Design review of the part built by this model. Coordinates are the model's own, in mm. Give positions to 0.01 mm unless a question says otherwise; leave off trailing zeros. Write each loop counter-clockwise with the first axis right and the second up, starting at its lowest first coordinate (ties: lowest second). Pieces come first, ordered by that corner, then holes. Notation, with made-up numbers: (-3.5, -24.75) -> (23.5, -24.75) arc R16 ccw to (23.5, -7.75) -> close; hole circle Ø3 at (17, 70.5). An arc over 180 degrees is marked (long way). Return JSON: item names as keys, results as strings. Group by question number.
from build123d import *

# Parameters (mm, degrees)
SKETCH1_W                       = 66.04
SKETCH1_H                       = 15.24
BOSS_EXTRUDE1_DEPTH             = 6
CBORE_FOR_M3_SBHCS1_D           = 3.6
CBORE_FOR_M3_SBHCS1_CBORE_D     = 6.7
CBORE_FOR_M3_SBHCS1_CBORE_DEPTH = 1.65
FILLET1_R                       = 5.08
FILLET2_R                       = 1.27


with BuildPart() as part:
    # Sketch1 → Boss-Extrude1 (new body)
    with BuildSketch(Plane(origin=(0, 0, 0), x_dir=(1, 0, 0), z_dir=(0, 1, 0))):
        with Locations((33.02, -7.62)):
            Rectangle(SKETCH1_W, SKETCH1_H)
    extrude(amount=BOSS_EXTRUDE1_DEPTH)

    # CBORE for M3 SBHCS1 (through all)
    with Locations(Plane(origin=(0, 6, 0), x_dir=(1, 0, 0), z_dir=(0, 1, 0))):
        with Locations((16.51, -7.62), (49.53, -7.62)):
            CounterBoreHole(CBORE_FOR_M3_SBHCS1_D / 2, CBORE_FOR_M3_SBHCS1_CBORE_D / 2, CBORE_FOR_M3_SBHCS1_CBORE_DEPTH)

    # Fillet1
    fillet1_edges = [part.edges().sort_by_distance(p)[0] for p in [
        (0, 3, 0),
        (66.04, 3, 0),
        (66.04, 3, 15.24),
        (0, 3, 15.24),
    ]]
    fillet(fillet1_edges, radius=FILLET1_R)

    # Fillet2
    fillet2_edges = [part.edges().sort_by_distance(p)[0] for p in [
        (33.02, 6, 15.24),
        (0, 6, 7.62),
        (66.04, 6, 7.62),
        (33.02, 6, 0),
        (64.552102448, 6, 1.487897552),
        (64.552102448, 6, 13.752102448),
        (1.487897552, 6, 1.487897552),
        (1.487897552, 6, 13.752102448),
    ]]
    fillet(fillet2_edges, radius=FILLET2_R)


solid = part.part
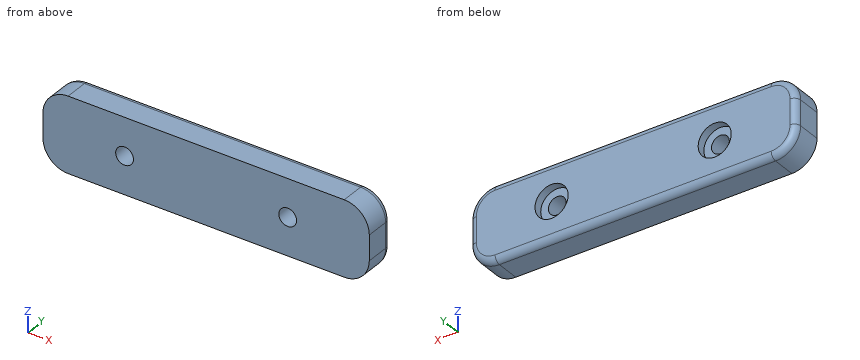
Q1. Take a section at B-B, the plane x = 49.53. Give the boundary of the cut face in (y, z), plus the area to 3 significant figures.
Q2. Insertion check: pin 1 (3.5 mm diameter, centred on x = 16.5, z = 9, fed in from +Y); pin 2 (1.5 mm diameter, centred on y = 2, z = 13.5, fed in from -X). Each pin has a flat end and moves straight along its axis. Give the tip position at first contact, or say it passes through.
Q3. For L1, parallel to X at y = 1.3, z = 7.62; L2, parallel to X at y = 5.6, z = 10; L3, parallel to Z at x = 49.53, y = 5, list the stretches that pass through material, from the lowest coordinate up. Write a range as from..to.
Q4. Take a section at A-A, the plane z = 7.62. Give the boundary of the cut face in (x, y).
Q5. Take a section at C-C, the plane y = 3.65. Give the boundary of the cut face in (x, z).
Final values:
{
 "1": {"outline": "(0, 0) -> (4.73, 0) arc R1.27 ccw to (6, 1.27) -> (6, 4.27) -> (4.35, 4.27) -> (4.35, 5.82) -> (0, 5.82) -> close; (0, 9.42) -> (4.35, 9.42) -> (4.35, 10.97) -> (6, 10.97) -> (6, 13.97) arc R1.27 ccw to (4.73, 15.24) -> (0, 15.24) -> close", "area": "64.0 mm²"},
 "2": {"pin 1": "stops at y = 4.35", "pin 2": "stops at x = 0.71"},
 "3": {"L1": "x = 0..14.71, 18.31..47.73, 51.33..66.04", "L2": "x = 0.34..14.15, 18.87..47.17, 51.89..65.7", "L3": "z = 0.03..4.27, 10.97..15.21"},
 "4": {"outline": "(0, 0) -> (14.71, 0) -> (14.71, 4.35) -> (13.16, 4.35) -> (13.16, 6) -> (1.27, 6) arc R1.27 ccw to (0, 4.73) -> close; (18.31, 0) -> (47.73, 0) -> (47.73, 4.35) -> (46.18, 4.35) -> (46.18, 6) -> (19.86, 6) -> (19.86, 4.35) -> (18.31, 4.35) -> close; (51.33, 0) -> (66.04, 0) -> (66.04, 4.73) arc R1.27 ccw to (64.77, 6) -> (52.88, 6) -> (52.88, 4.35) -> (51.33, 4.35) -> close"},
 "5": {"outline": "(0, 5.08) arc R5.08 ccw to (5.08, 0) -> (60.96, 0) arc R5.08 ccw to (66.04, 5.08) -> (66.04, 10.16) arc R5.08 ccw to (60.96, 15.24) -> (5.08, 15.24) arc R5.08 ccw to (0, 10.16) -> close; hole circle Ø3.6 at (16.51, 7.62); hole circle Ø3.6 at (49.53, 7.62)"}
}
